Geometry: see drawing. Coordinates: mm, zero at the bounding-box minimum. A direction names the side the tool comes from. Round coordinates to 2 decimals unless told otherwise and drop trailing zeros. Write each loop counter-clockwise with the first axis right and the second up, starting at its lowest first coordinate (ties: lowest second). Pieces come first, ordered by that corner, then holes. Notation, with made-up numbers: M -7.75,-27.75 L 3.25,-27.75 A25 cw 3.25,-3.75 Z; hole C 40,40.5 d8. An arc over 180 degrees is marked long. Use a Markdown table: item, result.
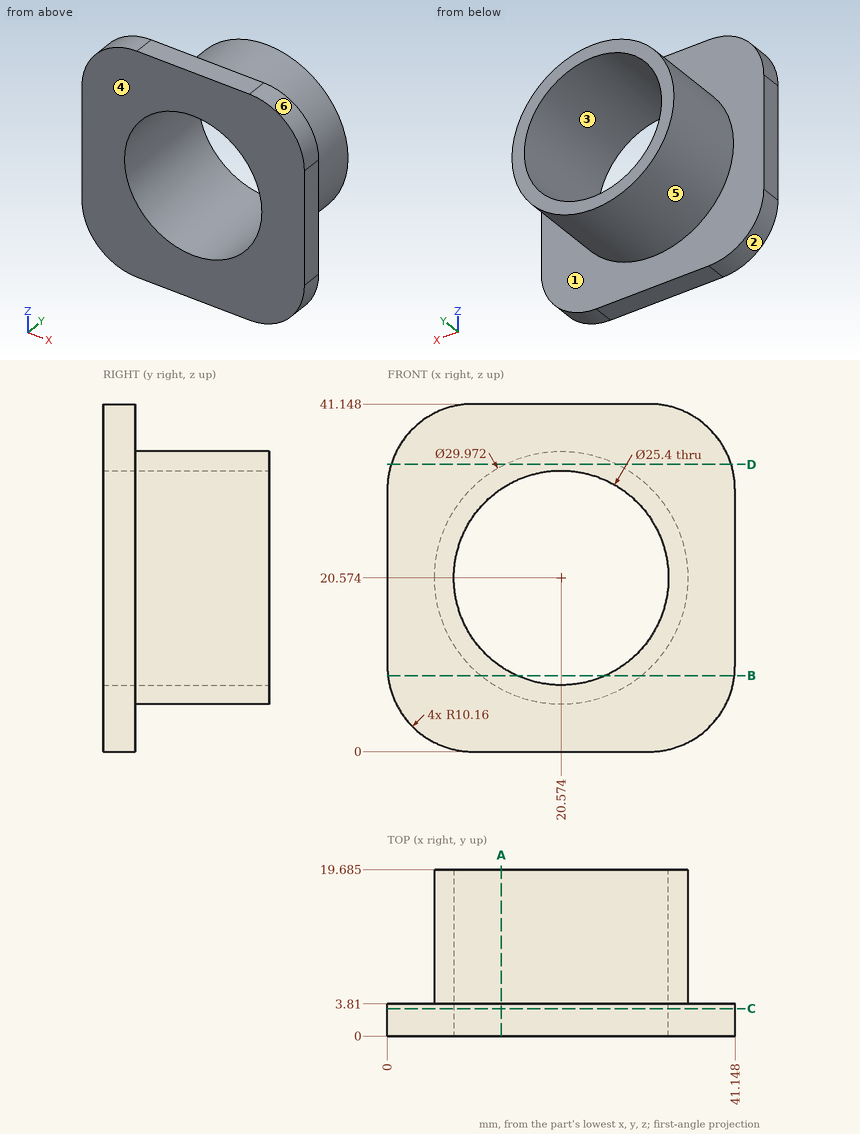
Q1. Reachability of the marked faces 1 and 2 from +Z, -Z, +X, -X, +Y, -Y: full face, straight path, thin tool, end or side. Return the list, or none.
Results are:
| item | result |
|---|---|
| face 1 | +Y |
| face 2 | -Z, -X, +Y, -Y |
Q2. Section B-B on z = 9. Return loops of the section in (x, y) (3 decimals), plus the area to 3 significant figures.
Results are:
| item | result |
|---|---|
| outline | M 0.066,0 L 15.346,0 L 15.346,19.685 L 11.054,19.685 L 11.054,3.81 L 0.066,3.81 Z; M 25.802,0 L 41.082,0 L 41.082,3.81 L 30.094,3.81 L 30.094,19.685 L 25.802,19.685 Z |
| area | 253 mm^2 |
Q3. Section C-C on y = 3.25. Return loops of the section in (x, z).
Results are:
| item | result |
|---|---|
| outline | M 0,10.16 A10.16 ccw 10.16,0 L 30.99,0 A10.16 ccw 41.15,10.16 L 41.15,30.99 A10.16 ccw 30.99,41.15 L 10.16,41.15 A10.16 ccw 0,30.99 Z; hole C 20.57,20.57 d25.4 |
Q4. Section A-A on x = 13.5. Return loops of the section in (y, z) (3 decimals), plus the area to 3 significant figures.
Results are:
| item | result |
|---|---|
| outline | M 0,0 L 3.81,0 L 3.81,7.363 L 19.685,7.363 L 19.685,10.027 L 0,10.027 Z; M 0,31.121 L 19.685,31.121 L 19.685,33.785 L 3.81,33.785 L 3.81,41.148 L 0,41.148 Z |
| area | 161 mm^2 |
Q5. Mould query, pull axis Z, two halves, no side actions, for the marked faces 3, 4, 5 and 6. Classes: +Z half, -Z half, draft (parallel to the pull), parting line (faces both ways), or undercut.
Results are:
| item | result |
|---|---|
| face 3 | undercut |
| face 4 | draft |
| face 5 | parting line |
| face 6 | +Z half |
Q6. Line query: L1, parallel to X at y = 6.25, z = 21; L2, parallel to Z at x = 20, y = 10.75; L3, parallel to Y at x = 38, z = 5.5. Output: solid intervals per line, ascending.
Results are:
| item | result |
|---|---|
| L1 | 5.59 to 7.88, 33.27 to 35.55 |
| L2 | 5.6 to 7.89, 33.26 to 35.55 |
| L3 | 0 to 3.81 |
Q7. Section D-D on z = 34. Return loops of the section in (x, y) (3 decimals).
Results are:
| item | result |
|---|---|
| outline | M 0.457,0 L 40.691,0 L 40.691,3.81 L 27.232,3.81 L 27.232,19.685 L 13.916,19.685 L 13.916,3.81 L 0.457,3.81 Z |
Q8. First-contact query: pin 1 Ø1 at (y, z) = (13.5, 6.5) entering from +X; pin 2 Ø1.5 at (x, y) = (25, 7.5) entering from +Z; pin 3 Ø1 at (y, z) = (5.5, 10) entering from -X. Flat tips, straight axial feed; report the tip coordinate or a pass-through.
Results are:
| item | result |
|---|---|
| pin 1 | x = 26.92 |
| pin 2 | z = 35.1 |
| pin 3 | x = 9.48 |
